```python
from build123d import *


with BuildPart() as f2:
    # F2: sweep along a path in F0
    with BuildLine(Plane.XZ) as f2_path:
        Line((300, 400), (-300, 400))
        Line((-300, 400), (-300, -400))
        Line((-300, -400), (300, -400))
        Line((300, -400), (300, 400))
    # F1 (on Top) → F2 (sweep)
    with BuildSketch(Plane.XY):
        with BuildLine():
            Line((-265, 0), (-300, 0))
            Line((-300, 0), (-300, -45))
            Line((-300, -45), (-263, -45))
            Line((-263, -45), (-263, -43))
            ThreePointArc((-263, -43), (-258.583592135, -37.7082039325), (-257, -31))
            Line((-257, -31), (-255, -31))
            Line((-255, -31), (-255, -15))
            Line((-255, -15), (-265, -15))
            Line((-265, -15), (-265, -11))
            Line((-265, -11), (-255, -11))
            Line((-255, -11), (-265, 0))
        make_face()
    sweep(path=f2_path.line, transition=Transition.RIGHT)


solid = f2.part
```
Geometry check sheet. Reference: the model listing, model coordinates, mm. A direction names the side the tool comes from. Give positions to 0.01 mm unless a question says otherwise; leave off trailing zeros. Write each loop counter-clockwise with the first axis right and the second up, starting at its lowest first coordinate (ties: lowest second). Pieces come first, ordered by that corner, then holes.
1) Section check A-A, the plane z = -333.5. Record the boundary of the cut face in (x, y), and give its area (3 significant figures).
2) Material ranges on L1, parallel to Z at x = -164, y = -13.5; L2, parallel to Z at x = 169, y = -32.5; L3, parallel to X at y = -20, z = -183.5, recorded low to high.
3) Release check for a two-part mould opening along X. For faces 4 (the flat face through (-300, -22, -6)), 5 (the flat face through (300, -22, 6)), 6 (the flat face through (-255, -23, -5)), 7 (the flat face through (265.3, 0, -31.5)) record: pulls with the +X half, pulls with the -X half, needs draft (parallel to the pull), parting line crosses it, or undercut.
4) Section check B-B, the plane x = -93. Record the boundary of the cut face in (y, z).
5) Access from +Z, -Z, +X, -X, +Y, -Y to the whole of each face (thin tool, end or side, straight path). Record for faces 1 (the flat face through (-256, -15, -2)), 2 (the flat face through (4, -23, -355)), 3 (the flat face through (265, -45, 31)).
Computed:
1. outline: (-300, -45) - (-263, -45) - (-263, -43) arc R15 ccw to (-257, -31) - (-255, -31) - (-255, -15) - (-265, -15) - (-265, -11) - (-255, -11) - (-265, 0) - (-300, 0) - close; (255, -31) - (257, -31) arc R15 ccw to (263, -43) - (263, -45) - (300, -45) - (300, 0) - (265, 0) - (255, -11) - (265, -11) - (265, -15) - (255, -15) - close
1. area: 3,740 mm2
2. L1: z = -400 to -365, 365 to 400
2. L2: z = -400 to -357.08, 357.08 to 400
2. L3: x = -300 to -255, 255 to 300
3. face 4: pulls with the -X half
3. face 5: pulls with the +X half
3. face 6: undercut
3. face 7: needs draft
4. outline: (-45, -400) - (0, -400) - (0, -365) - (-11, -355) - (-11, -365) - (-15, -365) - (-15, -355) - (-31, -355) - (-31, -357) arc R15 ccw to (-43, -363) - (-45, -363) - close; (-45, 363) - (-43, 363) arc R15 ccw to (-31, 357) - (-31, 355) - (-15, 355) - (-15, 365) - (-11, 365) - (-11, 355) - (0, 365) - (0, 400) - (-45, 400) - close
5. face 1: none
5. face 2: +Y, -Y
5. face 3: +Z, -Z, +X, -X, -Y
